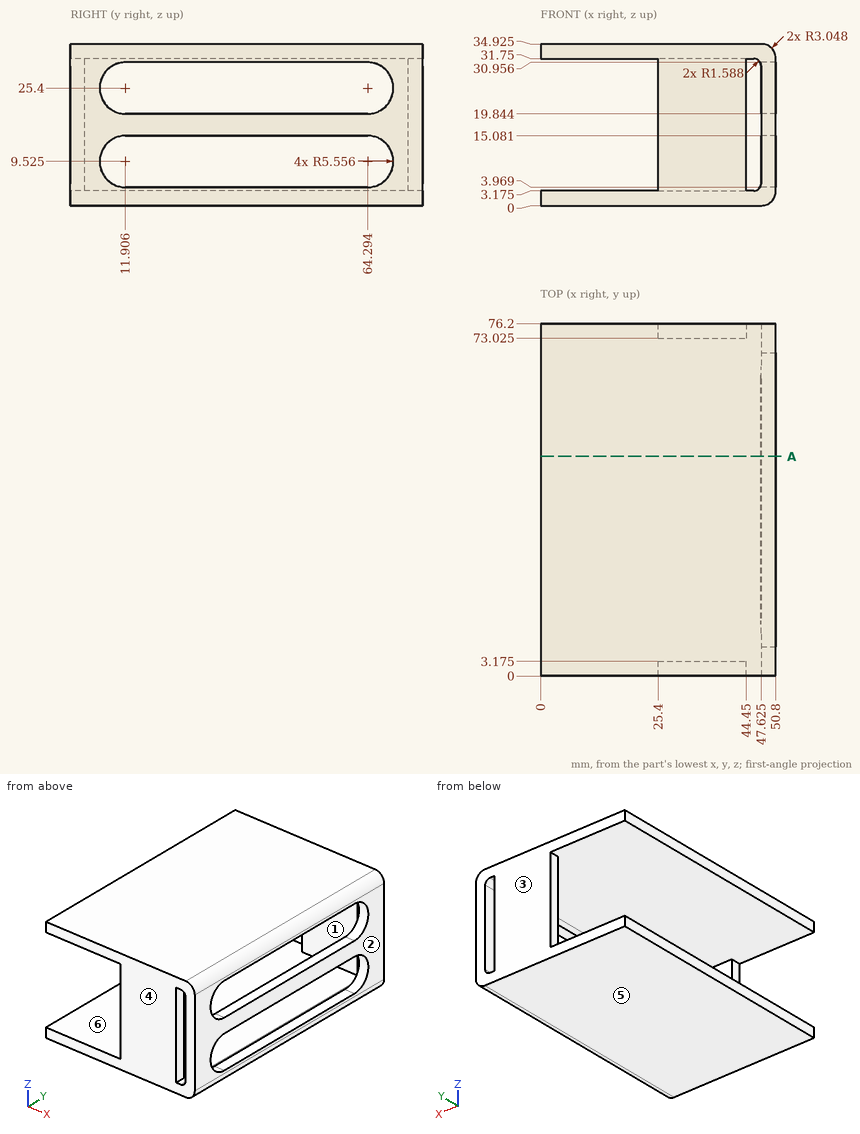
Geometry: see drawing. Coordinates: mm, zero at the bounding-box minimum. A direction names the side the tool comes from. Round coordinates to 2 decimals unless told otherwise and drop trailing zeros. Use a Markdown table: item, result. Add a question column.
1. Ray query, line 1 along Y through (x, z) = (29, 17.5) (1 decimal); line 2 along X through (y, z) = (5, 28) (1 decimal); line 3 along Y through (x, z) = (48.5, 12.5) (1 decimal). Return the intervals inside material, ascending. Write a range as [from, to].
2. Cut plane A-A, the plane y = 47.5. State how many separate pieces and enclosed holes the cut face has.
3. Pull-direction query (Y, two-part tool) for the marked faces 3, 4, 5 and 6; classes: +Y half, -Y half, draft (parallel to the pull), parting line (faces both ways), or undercut.
4. Set-up query: the marked faces 1 and 2. Return all of +Z, -Z, +X, -X, +Y, -Y with unobstructed straight access to the full face (end or side cutting, diameter ignored); none if empty.
5. Contact query for flat-ended pins moving along their axis: pin 1 (1.5 mm diameter, centred on x = 34.5, y = 49, fed in from -Z); pin 2 (1 mm diameter, centred on y = 1, z = 18, fed in from -X); pin 3 (3.5 mm diameter, centred on x = 50, y = 43, fed in from +Z); pin 4 (7.5 mm diameter, centred on y = 21.5, z = 19, fed in from -X) (1 decimal). Output: stop coordinate, or through.
Solution:
| question | item | result |
|---|---|---|
| 1 | line 1 | y = [0, 3.2], [73, 76.2] |
| 1 | line 2 | x = [47.6, 50.8] |
| 1 | line 3 | y = [0, 7.2], [69, 76.2] |
| 2 | separate pieces | 3 |
| 2 | enclosed holes | 0 |
| 3 | face 3 | +Y half |
| 3 | face 4 | -Y half |
| 3 | face 5 | draft |
| 3 | face 6 | undercut |
| 4 | face 1 | -X |
| 4 | face 2 | +Z, -Z, +X, +Y, -Y |
| 5 | pin 1 | stops at z = 0 |
| 5 | pin 2 | stops at x = 25.4 |
| 5 | pin 3 | stops at z = 34.88 |
| 5 | pin 4 | stops at x = 47.6 |
